Check sheet for the drawn part. Datum: minimum x, y, z corner. Units: mm. A direction names the side the tool comes from. Coordinates: 2 decimals unless noted, no trailing zeros. Write each loop counter-clockwise with the first axis right and the second up, starting at its lowest first coordinate (ties: lowest second). Pieces come first, ordered by that corner, then holes. Notation, with made-up numbers: (31.5, -1) -> (49.5, -1) arc R11 cw to (49.5, 14) -> close; hole circle Ø8 at (68, 46.5). An arc over 180 degrees is marked (long way). Answer in a Markdown table with one row per item.
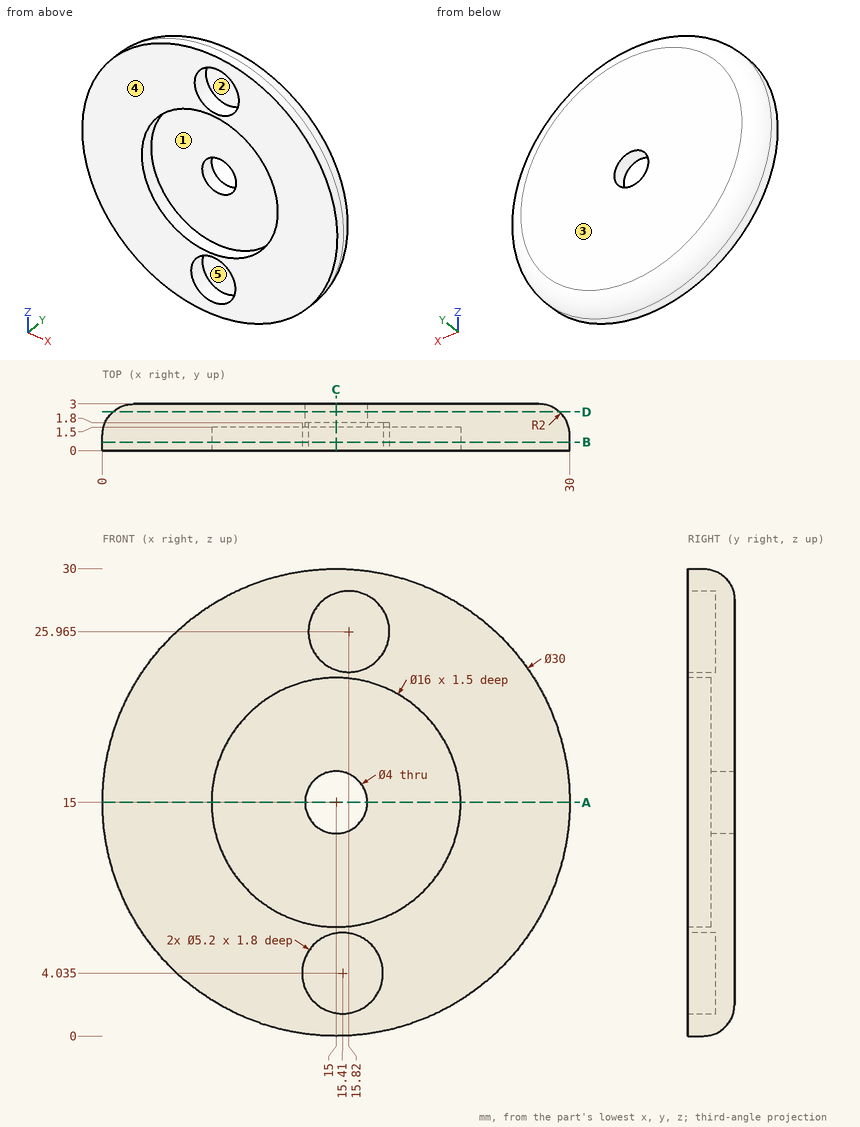
1. Release check for a two-part mould opening along X. For the marked faces 1, 2 and 3 record: released by +X, released by -X, zero draft, split by the parting line, or undercut.
Findings below:
| item | result |
|---|---|
| face 1 | undercut |
| face 2 | undercut |
| face 3 | zero draft |
2. Sectioned sample at C-C, the plane x = 15. Record the cut outline in (y, z), and give its area (3 significant figures).
Findings below:
| item | result |
|---|---|
| outline | (0, 0) -> (1, 0) arc R2 ccw to (3, 2) -> (3, 13) -> (1.5, 13) -> (1.5, 7) -> (0, 7) -> (0, 6.6) -> (1.8, 6.6) -> (1.8, 1.47) -> (0, 1.47) -> close; (0, 23) -> (1.5, 23) -> (1.5, 17) -> (3, 17) -> (3, 28) arc R2 ccw to (1, 30) -> (0, 30) -> (0, 28.43) -> (1.8, 28.43) -> (1.8, 23.5) -> (0, 23.5) -> close |
| area | 40.2 mm² |
3. Access from +Z, -Z, +X, -X, +Y, -Y to the whole of each face (thin tool, end or side, straight path). Record for the marked faces 4 and 5.
Findings below:
| item | result |
|---|---|
| face 4 | +Z, -Z, +X, -X, -Y |
| face 5 | -Y |
4. Go/stop test with flat-tipped pins: pin 1 (1.5 mm diameter, centred on x = 7.5, y = 0.5, fed in from +Z); pin 2 (1.6 mm diameter, centred on x = 14, z = 3, fed in from -Y); pin 3 (5 mm diameter, centred on x = 15.5, z = 16.5, fed in from -Y); pin 4 (2.5 mm diameter, centred on x = 15, z = 15, fed in from -Y). Record where each tip stops, or that it passes through.
Findings below:
| item | result |
|---|---|
| pin 1 | stops at z = 28.4 |
| pin 2 | stops at y = 1.8 |
| pin 3 | stops at y = 1.5 |
| pin 4 | passes through |
5. Sectioned sample at A-A, the plane z = 15. Record the cut outline in (x, y).
Findings below:
| item | result |
|---|---|
| outline | (0, 0) -> (7, 0) -> (7, 1.5) -> (13, 1.5) -> (13, 3) -> (2, 3) arc R2 ccw to (0, 1) -> close; (17, 1.5) -> (23, 1.5) -> (23, 0) -> (30, 0) -> (30, 1) arc R2 ccw to (28, 3) -> (17, 3) -> close |
6. Sectioned sample at D-D, the plane y = 2.5. Record the cut outline in (x, z), and give its area (3 significant figures).
Findings below:
| item | result |
|---|---|
| outline | circle Ø28.65 at (15, 15); hole circle Ø4 at (15, 15) |
| area | 632 mm² |
7. Sectioned sample at B-B, the plane y = 0.55. Record the cut outline in (x, z) (3 decimals), and give its area (3 significant figures).
Findings below:
| item | result |
|---|---|
| outline | circle Ø30 at (15, 15); hole circle Ø16 at (15, 15); hole circle Ø5.2 at (15.41, 4.035); hole circle Ø5.2 at (15.82, 25.965) |
| area | 463 mm² |
8. Material ranges on probe 1 along X at (y, z) = (0.75, 15); probe 2 along Z at (x, y) = (16, 1.65); probe 3 along Z at (x, y) = (14, 0.6), recorded low to high. Write a range as from..to.
Findings below:
| item | result |
|---|---|
| probe 1 | x = 0..7, 23..30 |
| probe 2 | z = 0.14..1.5, 6.57..13.27, 16.73..23.37, 28.56..29.86 |
| probe 3 | z = 0.03..1.85, 6.22..7.06, 22.94..24.11, 27.82..29.97 |
